Build history of the part. All positions in model axes, mm. A direction names the side the tool comes from. Round coordinates to 2 decimals unless told otherwise and drop trailing zeros. Write each loop counter-clockwise with the first axis right and the second up, starting at its lowest first coordinate (ties: lowest second). Pieces come first, ordered by that corner, then holes. Notation, with made-up numbers: M 24.25,48 L 52.25,48 A20 ccw 52.25,84 Z; hole C 28.25,-32.75 d3. An arc over 180 degrees is marked long. Use a Markdown table: item, result.
from build123d import *

# Parameters (mm, degrees)
SKETCH_2_R          = 1.1
SKETCH_2_R_2        = 2.25
SKETCH_2_W          = 25.8
SKETCH_2_H          = 2.4
SKETCH_2_W_2        = 20.6
SKETCH_2_W_3        = 18.2
EXTRUDE_1_DEPTH     = 3
CHAMFER_1_SIZE      = 1
SKETCH_3_W          = 26.8
SKETCH_3_H          = 3.4
SKETCH_3_W_2        = 19.2
SKETCH_3_W_3        = 21.6
CUT_EXTRUDE_1_DEPTH = 54.573406165
CHAMFER_2_SIZE      = 2
EXTRUDE_START       = -2.2
SKETCH_4_R          = 4
SKETCH_4_R_2        = 2.25
EXTRUDE_2_DEPTH     = 2.2
SKETCH_5_W          = 3
SKETCH_5_H          = 3
EXTRUDE_3_DEPTH     = 8.5
CHAMFER_3_SIZE      = 1
SKETCH_6_R          = 1.5
CUT_EXTRUDE_2_DEPTH = 55.160500811


with BuildPart() as part:
    # 草图2 → 凸台-拉伸1 (new body)
    with BuildSketch(Plane(origin=(0, 0, 0), x_dir=(1, 0, 0), z_dir=(0, 1, 0))):
        with BuildLine():
            Line((37.46902332, -26.75), (-37.46902332, -26.75))
            ThreePointArc((-37.46902332, -26.75), (-38.093655246, -26.969080697), (-38.444597576, -27.530330086))
            ThreePointArc((-38.444597576, -27.530330086), (-43.492640687, -28.992640687), (-42.030330086, -23.944597576))
            ThreePointArc((-42.030330086, -23.944597576), (-41.469080697, -23.593655246), (-41.25, -22.96902332))
            Line((-41.25, -22.96902332), (-41.25, 22.96902332))
            ThreePointArc((-41.25, 22.96902332), (-41.469080697, 23.593655246), (-42.030330086, 23.944597576))
            ThreePointArc((-42.030330086, 23.944597576), (-43.492640687, 28.992640687), (-38.444597576, 27.530330086))
            ThreePointArc((-38.444597576, 27.530330086), (-38.093655246, 26.969080697), (-37.46902332, 26.75))
            Line((-37.46902332, 26.75), (37.46902332, 26.75))
            ThreePointArc((37.46902332, 26.75), (38.093655246, 26.969080697), (38.444597576, 27.530330086))
            ThreePointArc((38.444597576, 27.530330086), (43.492640687, 28.992640687), (42.030330086, 23.944597576))
            ThreePointArc((42.030330086, 23.944597576), (41.469080697, 23.593655246), (41.25, 22.96902332))
            Line((41.25, 22.96902332), (41.25, -22.96902332))
            ThreePointArc((41.25, -22.96902332), (41.469080697, -23.593655246), (42.030330086, -23.944597576))
            ThreePointArc((42.030330086, -23.944597576), (43.492640687, -28.992640687), (38.444597576, -27.530330086))
            ThreePointArc((38.444597576, -27.530330086), (38.093655246, -26.969080697), (37.46902332, -26.75))
        make_face()
        with Locations(Location((-41.371320344, 26.871320344, 0), (0, 0, 270))):
            Circle(SKETCH_2_R, mode=Mode.SUBTRACT)
        with Locations(Location((-41.371320344, -26.871320344, 0), (0, 0, 270))):
            Circle(SKETCH_2_R, mode=Mode.SUBTRACT)
        with Locations(Location((41.371320344, -26.871320344, 0), (0, 0, 270))):
            Circle(SKETCH_2_R, mode=Mode.SUBTRACT)
        with Locations(Location((41.371320344, 26.871320344, 0), (0, 0, 270))):
            Circle(SKETCH_2_R, mode=Mode.SUBTRACT)
        with Locations(Location((0, 20, 0), (0, 0, 270))):
            Circle(SKETCH_2_R_2, mode=Mode.SUBTRACT)
        with Locations(Location((-20, -20, 0), (0, 0, 270))):
            Circle(SKETCH_2_R_2, mode=Mode.SUBTRACT)
        with Locations(Location((20, -20, 0), (0, 0, 270))):
            Circle(SKETCH_2_R_2, mode=Mode.SUBTRACT)
        with Locations((-19.1, 12.3)):
            Rectangle(SKETCH_2_W, SKETCH_2_H, mode=Mode.SUBTRACT)
        with Locations((18.9, 12.3)):
            Rectangle(SKETCH_2_W, SKETCH_2_H, mode=Mode.SUBTRACT)
        with Locations((-21.7, -12.3)):
            Rectangle(SKETCH_2_W_2, SKETCH_2_H, mode=Mode.SUBTRACT)
        with Locations((22.6, -12.3)):
            Rectangle(SKETCH_2_W_3, SKETCH_2_H, mode=Mode.SUBTRACT)
    extrude(amount=EXTRUDE_1_DEPTH)

    # 倒角1
    chamfer_1_edges = [part.edges().sort_by_distance(p)[0] for p in [
        (-41.371320344, 3, -27.971320344),
        (-41.371320344, 3, 25.771320344),
        (41.371320344, 3, 25.771320344),
        (41.371320344, 3, -27.971320344),
    ]]
    chamfer(chamfer_1_edges, length=CHAMFER_1_SIZE)

    # 草图3 → 切除-拉伸1 (cut, through all)
    with BuildSketch(Plane(origin=(0, 0, 0), x_dir=(1, 0, 0), z_dir=(0, 1, 0))):
        with Locations((-19.1, 12.3)):
            Rectangle(SKETCH_3_W, SKETCH_3_H)
        with Locations((18.9, 12.3)):
            Rectangle(SKETCH_3_W, SKETCH_3_H)
        with Locations((22.6, -12.3)):
            Rectangle(SKETCH_3_W_2, SKETCH_3_H)
        with Locations((-21.7, -12.3)):
            Rectangle(SKETCH_3_W_3, SKETCH_3_H)
    extrude(amount=CUT_EXTRUDE_1_DEPTH, mode=Mode.SUBTRACT)

    # 倒角2
    chamfer_2_edges = [part.edges().sort_by_distance(p)[0] for p in [
        (0, 3, -22.25),
        (-20, 3, 17.75),
        (20, 3, 17.75),
    ]]
    chamfer(chamfer_2_edges, length=CHAMFER_2_SIZE)

    # 草图4 → 凸台-拉伸2 (add)
    # profile 1 of 3: a face of its own
    with BuildSketch(Plane(origin=(0, 0, 0), x_dir=(1, 0, 0), z_dir=(0, 1, 0)).offset(EXTRUDE_START)):
        with Locations(Location((-20, -20, 0), (0, 0, 270))):
            Circle(SKETCH_4_R)
        with Locations(Location((-20, -20, 0), (0, 0, 270))):
            Circle(SKETCH_4_R_2, mode=Mode.SUBTRACT)
    # profile 2 of 3: a face of its own
    with BuildSketch(Plane(origin=(0, 0, 0), x_dir=(1, 0, 0), z_dir=(0, 1, 0)).offset(EXTRUDE_START)):
        with Locations(Location((20, -20, 0), (0, 0, 270))):
            Circle(SKETCH_4_R)
        with Locations(Location((20, -20, 0), (0, 0, 270))):
            Circle(SKETCH_4_R_2, mode=Mode.SUBTRACT)
    # profile 3 of 3: a face of its own
    with BuildSketch(Plane(origin=(0, 0, 0), x_dir=(1, 0, 0), z_dir=(0, 1, 0)).offset(EXTRUDE_START)):
        with Locations(Location((0, 20, 0), (0, 0, 270))):
            Circle(SKETCH_4_R)
        with Locations(Location((0, 20, 0), (0, 0, 270))):
            Circle(SKETCH_4_R_2, mode=Mode.SUBTRACT)
    extrude(amount=EXTRUDE_2_DEPTH)

    # 草图5 → 凸台-拉伸3 (add)
    with BuildSketch(Plane(origin=(0, 0, 0), x_dir=(1, 0, 0), z_dir=(0, 1, 0))):
        with Locations((37.5, 23)):
            Rectangle(SKETCH_5_W, SKETCH_5_H)
        with Locations((-37.5, 23)):
            Rectangle(SKETCH_5_W, SKETCH_5_H)
        with Locations((37.5, -23)):
            Rectangle(SKETCH_5_W, SKETCH_5_H)
        with Locations((-37.5, -23)):
            Rectangle(SKETCH_5_W, SKETCH_5_H)
    extrude(amount=-EXTRUDE_3_DEPTH)

    # 倒角3
    chamfer_3_edges = [part.edges().sort_by_distance(p)[0] for p in [
        (-37.5, 0, -21.5),
        (-36, 0, -23),
        (36, 0, -23),
        (37.5, 0, -21.5),
        (37.5, 0, 21.5),
        (36, 0, 23),
        (-36, 0, 23),
        (-37.5, 0, 21.5),
    ]]
    chamfer(chamfer_3_edges, length=CHAMFER_3_SIZE)

    # 草图6 → 切除-拉伸2 (cut, through all)
    with BuildSketch(Plane(origin=(0, 0, 0), x_dir=(1, 0, 0), z_dir=(0, 1, 0))):
        with Locations(Location((-35, -19, 0), (0, 0, 270))):
            Circle(SKETCH_6_R)
        with Locations(Location((35, -19, 0), (0, 0, 270))):
            Circle(SKETCH_6_R)
    extrude(amount=CUT_EXTRUDE_2_DEPTH, mode=Mode.SUBTRACT)


solid = part.part
Q1. Cut at B-B on y = -3.25. Give the cut face in (x, z), and give its area (3 significant figures).
Response values:
| item | result |
|---|---|
| outline | M -39,-24.5 L -36,-24.5 L -36,-21.5 L -39,-21.5 Z; M -39,21.5 L -36,21.5 L -36,24.5 L -39,24.5 Z; M 36,-24.5 L 39,-24.5 L 39,-21.5 L 36,-21.5 Z; M 36,21.5 L 39,21.5 L 39,24.5 L 36,24.5 Z |
| area | 36.0 mm2 |
Q2. Drill centre lines: L1, parallel to Z at x = -30.5, y = 1; L2, parallel to Z at x = 35, y = 0.75; L3, parallel to X at y = -1.5, z = -20. Where is each one in solid material? Low to high.
Response values:
| item | result |
|---|---|
| L1 | z = -26.75 to -14, -10.6 to 10.6, 14 to 26.75 |
| L2 | z = -26.75 to 17.5, 20.5 to 26.75 |
| L3 | x = -4 to -2.25, 2.25 to 4 |
Q3. Cut at D-D on x = -30. Give the cut face in (y, z).
Response values:
| item | result |
|---|---|
| outline | M 0,-26.75 L 3,-26.75 L 3,-14 L 0,-14 Z; M 0,-10.6 L 3,-10.6 L 3,10.6 L 0,10.6 Z; M 0,14 L 3,14 L 3,26.75 L 0,26.75 Z |
Q4. Cut at A-A on z = 12.5. Give the cut face in (x, y), and give its area (3 significant figures).
Response values:
| item | result |
|---|---|
| outline | M -41.25,0 L -32.5,0 L -32.5,3 L -41.25,3 Z; M -10.9,0 L 13,0 L 13,3 L -10.9,3 Z; M 32.2,0 L 41.25,0 L 41.25,3 L 32.2,3 Z |
| area | 125 mm2 |
Q5. Cut at C-C on x = 0. Give the cut face in (y, z), and give its area (3 significant figures).
Response values:
| item | result |
|---|---|
| outline | M -2.2,-24 L 0,-24 L 0,-26.75 L 3,-26.75 L 3,-24.25 L 1,-22.25 L -2.2,-22.25 Z; M -2.2,-17.75 L 1,-17.75 L 3,-15.75 L 3,26.75 L 0,26.75 L 0,-16 L -2.2,-16 Z |
| area | 151 mm2 |
Q6. Two-plate mould, pull along Z, no slides. Class faces 6 (the cylindrical face through (43.555, 1.479, 28.928)), 7 (the flat face through (37, -8.5, -23)): +Z half, -Z half, draft (parallel to the pull), parting line (faces both ways), or undercut.
Response values:
| item | result |
|---|---|
| face 6 | undercut |
| face 7 | draft |
Q7. Drop flat-ended pins along their axis: P1, Ø5, axis at y = -6.5, z = 14.5, coming from the -X side; P2, Ø3.5, axis at y = 1, z = -12.5, coming from the -X side; P3, Ø0.9, axis at x = 4, y = 1, coming from the +Z side; P4, Ø0.9, axis at x = 16.5, y = 1.5, coming from the -Z side. Give the stop position or say it passes through.
Response values:
| item | result |
|---|---|
| P1 | passes through |
| P2 | stops at x = -41.25 |
| P3 | stops at z = 26.75 |
| P4 | stops at z = -26.75 |
Q8. Which spindle directions (+Z, -Z, +X, -X, +Y, -Y) get a long thin tool onto all of the face, cutting with end or side? Do faces 1 (the flat face through (-41.25, 1, 0)), 2 (the flat face through (39, -4, -23)), 3 (the flat face through (-32.5, 1, 12)), 4 (the flat face through (37, -5, -21.5)), 5 (the flat face through (-39, -4, 23)). Say none if no direction does.
Response values:
| item | result |
|---|---|
| face 1 | -X, +Y, -Y |
| face 2 | +Z, -Z, +X, -Y |
| face 3 | +Y, -Y |
| face 4 | +X, -Y |
| face 5 | +Z, -Z, -X, -Y |
